```python
from build123d import *

# Parameters (mm, degrees)
SKETCH1_R           = 10
BOSS_EXTRUDE1_DEPTH = 66.666666667
SCALE_1_SCALE       = 0.3
SKETCH_1_R          = 6
EXTRUDE_1_DEPTH     = 3
SKETCH_2_R          = 3
SKETCH_2_R_2        = 2.75
CUT_EXTRUDE_1_DEPTH = 20


with BuildPart() as part:
    # Sketch1 → Boss-Extrude1 (new body)
    with BuildSketch(Plane(origin=(0, 0, 0), x_dir=(1, 0, 0), z_dir=(0, 1, 0))):
        Circle(SKETCH1_R)
    extrude(amount=BOSS_EXTRUDE1_DEPTH)


with BuildPart() as part_1:
    # 축척1: scaled about (0, 33.333333333, 0)
    add(part.part.scale(SCALE_1_SCALE).moved(Location((0, 23.333333333, 0))))

    # 스케치1 → 보스-돌출1 (add)
    with BuildSketch(Plane(origin=(0, 43.333333333, 0), x_dir=(1, 0, 0), z_dir=(0, 1, 0))):
        Circle(SKETCH_1_R)
    extrude(amount=EXTRUDE_1_DEPTH)

    # 스케치2 → 컷-돌출1 (cut)
    with BuildSketch(Plane.XZ.offset(-23.333333333)):
        Circle(SKETCH_2_R)
        Circle(SKETCH_2_R_2, mode=Mode.SUBTRACT)
    extrude(amount=-CUT_EXTRUDE_1_DEPTH, mode=Mode.SUBTRACT)


solid = part_1.part
```
Input: part model. Units: mm. Frame: model coordinates. A direction names the side the tool comes from. Coordinates: 2 decimals unless noted, no trailing zeros. Loops run counter-clockwise (first coordinate to the right, second up) from the corner with the lowest first, then second, coordinate; pieces in that order, holes last. Notation, with made-up numbers: M 13.5,-26.75 L 43.5,-26.75 A16 ccw 43.5,-5.75 Z; hole C 86,45.5 d4. An arc over 180 degrees is marked long. Answer in a Markdown table with one row per item.
1. Section B-B, the plane z = 0. Output: boundary loops of the cut face in (x, y), then the cut area to 3 significant figures.
Response:
| item | result |
|---|---|
| outline | M -6,43.33 L -2.75,43.33 L -2.75,23.33 L 2.75,23.33 L 2.75,43.33 L 6,43.33 L 6,46.33 L -6,46.33 Z |
| area | 146 mm2 |
2. First-contact query: pin 1 (1 mm diameter, centred on y = 38, z = 1.5, fed in from +X); pin 2 (1.5 mm diameter, centred on x = -4, y = 27.5, fed in from -Z). Flat tips, straight axial feed; report the tip coordinate or a pass-through.
Response:
| item | result |
|---|---|
| pin 1 | stops at x = 2.56 |
| pin 2 | passes through |
3. Reachability of faces 1 (the flat face through (0, 46.333, 0)), 2 (the flat face through (3, 43.333, 1)) from +Z, -Z, +X, -X, +Y, -Y: full face, straight path, thin tool, end or side. Return the list, or none.
Response:
| item | result |
|---|---|
| face 1 | +Z, -Z, +X, -X, +Y |
| face 2 | -Y |
4. Material intervals for line 1 (Y direction, x = -4, z = 1.75); line 2 (Z direction, x = 2, y = 35.5); line 3 (Z direction, x = -1.25, y = 41.5), sorted ascending.
Response:
| item | result |
|---|---|
| line 1 | y = 43.33 to 46.33 |
| line 2 | z = -1.89 to 1.89 |
| line 3 | z = -2.45 to 2.45 |
5. Section C-C, the plane y = 44. Output: boundary loops of the cut face in (x, z).
Response:
| item | result |
|---|---|
| outline | C 0,0 d12 |
6. Section D-D, the plane x = -3.25. Output: boundary loops of the cut face in (y, z).
Response:
| item | result |
|---|---|
| outline | M 43.33,-5.04 L 46.33,-5.04 L 46.33,5.04 L 43.33,5.04 Z |
7. Section A-A, the plane x = 0. Output: boundary loops of the cut face in (y, z).
Response:
| item | result |
|---|---|
| outline | M 23.33,-2.75 L 43.33,-2.75 L 43.33,-6 L 46.33,-6 L 46.33,6 L 43.33,6 L 43.33,2.75 L 23.33,2.75 Z |
8. Draft query along Z for faces 3 (the cylindrical face through (-0.596, 33.193, -2.685)), 4 (the flat face through (0, 23.333, 0)). Return one class per face: pulls with the +Z half, pulls with the -Z half, needs draft (parallel to the pull), parting line crosses it, or undercut.
Response:
| item | result |
|---|---|
| face 3 | parting line crosses it |
| face 4 | needs draft |
